from build123d import *

# Parameters (mm, degrees)
ESQUISSE1_R        = 3
BOSS_EXTRU_1_DEPTH = 2
CONG_1_R           = 18
CONG_2_R           = 20
D_GAGEMENT_M31_D   = 3.4


with BuildPart() as part:
    # Esquisse1 → Boss.-Extru.1 (new body)
    with BuildSketch(Plane.XY):
        Polygon((-244.958991582, 40), (-110, 40), (110, 40), (244.958991582, 40), (112.479495791, -30), (-112.479495791, -30), align=None)
        with Locations((-175, 20)):
            Circle(ESQUISSE1_R, mode=Mode.SUBTRACT)
        with Locations((-110, -20)):
            Circle(ESQUISSE1_R, mode=Mode.SUBTRACT)
        with Locations((110, -20)):
            Circle(ESQUISSE1_R, mode=Mode.SUBTRACT)
        with Locations((175, 20)):
            Circle(ESQUISSE1_R, mode=Mode.SUBTRACT)
        with Locations((0, -20)):
            Circle(ESQUISSE1_R, mode=Mode.SUBTRACT)
        with Locations((-58.333333333, 20)):
            Circle(ESQUISSE1_R, mode=Mode.SUBTRACT)
        with Locations((58.333333333, 20)):
            Circle(ESQUISSE1_R, mode=Mode.SUBTRACT)
    extrude(amount=BOSS_EXTRU_1_DEPTH)

    # Congé1
    cong_1_edges = [part.edges().sort_by_distance(p)[0] for p in [
        (-244.958991582, 40, 1),
        (244.958991582, 40, 1),
    ]]
    fillet(cong_1_edges, radius=CONG_1_R)

    # Congé2
    cong_2_edges = [part.edges().sort_by_distance(p)[0] for p in [
        (112.479495791, -30, 1),
        (-112.479495791, -30, 1),
    ]]
    fillet(cong_2_edges, radius=CONG_2_R)

    # Dégagement M31 (through all)
    with Locations(Plane(origin=(0, 0, 0), x_dir=(-1, 0, 0), z_dir=(0, 0, -1))):
        with Locations((160, 33.228756555), (175, 12.5), (160, 6.771243445)):
            Hole(D_GAGEMENT_M31_D / 2)


solid = part.part
Here's how the part is built. I have some questions about the finished solid (model axes, mm). Round coordinates to 2 decimals unless told otherwise and drop trailing zeros. Order: outer loops, then holes, each group sorted by start corner. A loop starts at its lowest first (then second) coordinate and runs counter-clockwise, first axis right, second up. Notation, with made-up numbers: M -21.5,64.5 L -5.5,64.5 A25 ccw -5.5,102.5 Z; hole C 58.25,29.25 d11. An arc over 180 degrees is marked long. Return JSON: item names as keys, results as strings. Group by question number.
1. I'm going to push a flat-ended pin straight in: pin 1 Ø3 at (x, y) = (-160, 33.23) entering from -Z (1 decimal). Where does the tip first touch, or does it pass through?
2. Please list where these lines run through material, in increasing order: probe 1 along X at (y, z) = (-21, 0.55); probe 2 along X at (y, z) = (21.5, 1.1); probe 3 along X at (y, z) = (21, 1.7).
3. If we section it at B-B on x = 166.5: List the corners of the cut face in (y, z) for me, then the cut area to 3 significant figures.
4. If we section it at C-C on y = -4: List the corners of the cut face in (x, z) for me.
5. If we mould it in two halves opening along X, with no side actions, what happens to faces 1 (the face through (-107.23, -21.15, 0.99)), 2 (the face through (149.27, -10.56, 0.99)), 3 (the face through (-148.371, -11.035, 0.986))? For each: pulls with the +X half, pulls with the -X half, needs draft (parallel to the pull), parting line crosses it, or undercut.
6. If we section it at A-A on z = 1.1: State how many separate pieces and enclosed holes the cut face has, then the cut area to 3 significant figures.
Reply:
{
 "1": {"pin 1": "through"},
 "2": {"probe 1": "-129.51 to -112.83, -107.17 to -2.83, 2.83 to 107.17, 112.83 to 129.51", "probe 2": "-190.36 to -177.6, -172.4 to -60.93, -55.74 to 55.74, 60.93 to 172.4, 177.6 to 190.36", "probe 3": "-190.34 to -177.83, -172.17 to -61.16, -55.5 to 55.5, 61.16 to 172.17, 177.83 to 190.34"},
 "3": {"outline": "M -1.46,0 L 40,0 L 40,2 L -1.46,2 Z", "area": "82.9 mm^2"},
 "4": {"outline": "M -161.69,0 L 161.69,0 L 161.69,2 L -161.69,2 Z"},
 "5": {"face 1": "undercut", "face 2": "pulls with the +X half", "face 3": "pulls with the -X half"},
 "6": {"separate pieces": "1", "enclosed holes": "10", "area": "23,000 mm^2"}
}
